Verification items for this drawing (mm, ordinates from the low corner). A direction names the side the tool comes from. Round coordinates to 2 decimals unless told otherwise and drop trailing zeros. Order: outer loops, then holes, each group sorted by start corner. A loop starts at its lowest first (then second) coordinate and runs counter-clockwise, first axis right, second up. Notation, with made-up numbers: (42, 32) -> (55, 32) arc R3 ccw to (55, 36) -> close; hole circle Ø5 at (81.5, 29). An arc over 180 degrees is marked (long way). Answer in a Markdown table with one row per item.
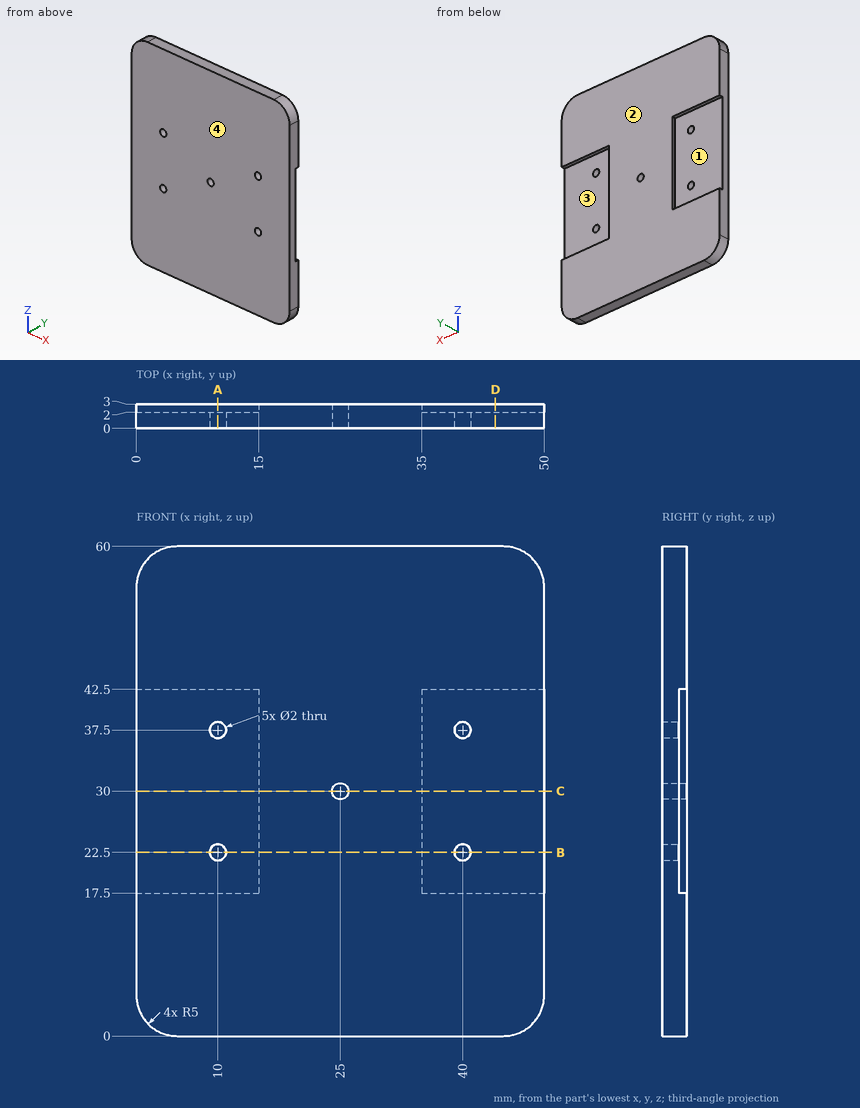
Item 1: Cross-section at A-A (x = 10). Record the boundary of the cut face in (y, z), and give its area (3 significant figures).
Result sheet:
| item | result |
|---|---|
| outline | (0, 0) -> (3, 0) -> (3, 17.5) -> (2, 17.5) -> (2, 21.5) -> (0, 21.5) -> close; (0, 23.5) -> (2, 23.5) -> (2, 36.5) -> (0, 36.5) -> close; (0, 38.5) -> (2, 38.5) -> (2, 42.5) -> (3, 42.5) -> (3, 60) -> (0, 60) -> close |
| area | 147 mm^2 |
Item 2: Cross-section at D-D (x = 44). Record the boundary of the cut face in (y, z).
Result sheet:
| item | result |
|---|---|
| outline | (0, 0) -> (3, 0) -> (3, 17.5) -> (2, 17.5) -> (2, 42.5) -> (3, 42.5) -> (3, 60) -> (0, 60) -> close |
Item 3: Cross-section at C-C (z = 30). Record the boundary of the cut face in (x, y).
Result sheet:
| item | result |
|---|---|
| outline | (0, 0) -> (24, 0) -> (24, 3) -> (15, 3) -> (15, 2) -> (0, 2) -> close; (26, 0) -> (50, 0) -> (50, 2) -> (35, 2) -> (35, 3) -> (26, 3) -> close |
Item 4: Set-up check for the marked faces 3 and 4: record each of +Z, -Z, +X, -X, +Y, -Y from which the full face is reachable in a straight line by a thin tool's end or side.
Result sheet:
| item | result |
|---|---|
| face 3 | +X, +Y |
| face 4 | +Z, -Z, +X, -X, -Y |
Item 5: Mould release check, pull along Z, two halves, no side actions. Record for the marked faces 1 and 2: pulls with the +Z half, pulls with the -Z half, needs draft (parallel to the pull), parting line crosses it, or undercut.
Result sheet:
| item | result |
|---|---|
| face 1 | undercut |
| face 2 | needs draft |
Item 6: Cross-section at B-B (z = 22.5). Record the boundary of the cut face in (x, y).
Result sheet:
| item | result |
|---|---|
| outline | (0, 0) -> (9, 0) -> (9, 2) -> (0, 2) -> close; (11, 0) -> (39, 0) -> (39, 2) -> (35, 2) -> (35, 3) -> (15, 3) -> (15, 2) -> (11, 2) -> close; (41, 0) -> (50, 0) -> (50, 2) -> (41, 2) -> close |
Item 7: Scan lines: line 1 (X direction, y = 0.45, z = 22.5); line 2 (Z direction, x = 10, y = 0.85); line 3 (Z direction, x = 43, y = 2.2). Record each from-to range of solid material in increasing order. Write a range as [from, to].
Result sheet:
| item | result |
|---|---|
| line 1 | x = [0, 9], [11, 39], [41, 50] |
| line 2 | z = [0, 21.5], [23.5, 36.5], [38.5, 60] |
| line 3 | z = [0, 17.5], [42.5, 60] |
Item 8: Depth check by flat-ended pin: P1, Ø0.5, axis at x = 4.5, y = 2.5, coming from the +Z side; P2, Ø0.8, axis at y = 2.5, z = 34, coming from the +X side; P3, Ø2.5, axis at x = 10, z = 22.5, coming from the +Y side; P4, Ø1.8, axis at x = 25, z = 30, coming from the +Y side. Enter the tip coordinate at first touch or a pass-through.
Result sheet:
| item | result |
|---|---|
| P1 | stops at z = 59.99 |
| P2 | stops at x = 35 |
| P3 | stops at y = 2 |
| P4 | passes through |
